from build123d import *

# Parameters (mm, degrees)
F0_R     = 3.56
F1_DEPTH = 14
F2_R     = 1
F3_DEPTH = 20.5
F5_DEPTH = 14
F6_COUNT = 10


with BuildPart() as f1:
    # F0 (on Top) → F1 (new body)
    with BuildSketch(Plane.XY):
        Circle(F0_R)
    extrude(amount=F1_DEPTH)

    # F2 (on face) → F3 (cut)
    with BuildSketch(Plane.XY.offset(14)):
        Circle(F2_R)
    extrude(amount=-F3_DEPTH, mode=Mode.SUBTRACT)

    # F4 (on face) → F5 (cut)
    with BuildSketch(Plane.XY.offset(14)):
        with BuildLine():
            ThreePointArc((-0.3510643437, 2.9307105578), (-0.2410218301, 2.6619758494), (0, 2.5))
            ThreePointArc((0, 2.5), (0.2410218301, 2.6619758494), (0.3510643437, 2.9307105578))
            Line((0.3510643437, 2.9307105578), (0.8662797764, 3.4529928104))
            ThreePointArc((0.8662797764, 3.4529928104), (0, 3.56), (-0.8662797764, 3.4529928104))
            Line((-0.8662797764, 3.4529928104), (-0.3510643437, 2.9307105578))
        make_face()
    f5 = extrude(amount=-F5_DEPTH, mode=Mode.SUBTRACT)

    # F6: F5 ×10 about axis
    f6_axis = Axis((0, 0, 0), (0, 0, -1))
    for i in range(1, F6_COUNT):
        add(f5.rotate(f6_axis, i * 360 / F6_COUNT), mode=Mode.SUBTRACT)


solid = f1.part
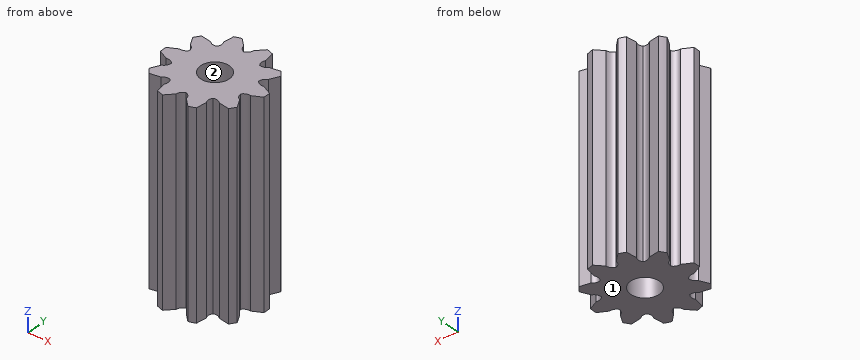
Geometry: final body of the model. Coordinates: model frame, mm. Face numbers are marked on the shaded views. Give positions to 0.01 mm unless a question says otherwise; leave off trailing zeros. Loops run counter-clockwise (first coordinate to the right, second up) from the corner with the lowest first, then second, coordinate; pieces in that order, holes last. Notation, with made-up numbers: M 45,71 L 60,71 A27 ccw 60,101 Z; hole C -32,80 d3. An arc over 180 degrees is marked long. Put each result on its own line as item: value.
1) Cut plane A-A, the plane y = 0. Return the cut outline in (x, z), plus the area to 3 significant figures.
Computed values:
outline: M -3.56,0 L -1,0 L -1,14 L -3.56,14 Z; M 1,0 L 3.56,0 L 3.56,14 L 1,14 Z
area: 71.7 mm^2
2) Cut plane B-B, the plane y = -1.75. Return the cut outline in (x, z), plus the area to 3 significant figures.
Computed values:
outline: M -2.94,0 L 2.94,0 L 2.94,14 L -2.94,14 Z
area: 82.4 mm^2
3) Material intervals for L1, parallel to X at y = 3.25, z = 4.5; L2, parallel to Y at x = 2.75, z = 3.5; L3, parallel to Y at x = -0.5, z = 4, sorted ascending. Write a range as from..to.
Computed values:
L1: x = -1.34..-0.67, 0.67..1.34
L2: y = -2.26..-1.38, -0.56..0.56, 1.38..2.26
L3: y = -3.08..-0.87, 0.87..3.08
4) Mould query, pull axis Y, two halves, no side actions, for the marked faces 1 and 2. Classes: released by +Y, released by -Y, zero draft, split by the parting line, or undercut.
Computed values:
face 1: zero draft
face 2: undercut
5) First-contact query: P1, Ø3, axis at x = -1.5, z = 12, coming from the -Y side. Flat tip, straight axial feed; report the tip coordinate or a pass-through.
Computed values:
P1: stops at y = -3.45
